Read the model definition and answer for the solid it produces. Units are mm, in the model's axes. A direction names the side the tool comes from. Coordinates: 2 decimals unless noted, no trailing zeros. Loops run counter-clockwise (first coordinate to the right, second up) from the corner with the lowest first, then second, coordinate; pieces in that order, holes last. Notation, with made-up numbers: (-5, 34.25) - (32, 34.25) arc R17 cw to (32, 62.25) - close; hole circle Ø3 at (18, 8.5). An arc over 180 degrees is marked (long way). One line per item, written item: value. Start each with the question number.
Autodesk Inventor part; units mm, degrees
ref_plane "YZ Plane" through (0, 0, 0) normal (1, 0, 0) x (0, 1, 0)
ref_plane "XZ Plane" through (0, 0, 0) normal (0, 1, 0) x (-1, 0, 0)
ref_plane "XY Plane" through (0, 0, 0) normal (0, 0, 1) x (1, 0, 0)
sketch "Sketch1" plane through (0, 0, 0) normal (0, 1, 0) x (-1, 0, 0)
  line L0 (50, 0) -> (0, 0)
  line L1 (0, 0) -> (0, -20)
  line L2 (0, -20) -> (50, -20)
  line L3 (50, -20) -> (50, 0)
  line L4 (0, 0) -> (20, 0)
  line L5 (20, 0) -> (20, -80)
  line L6 (20, -80) -> (0, -80)
  line L7 (0, -80) -> (0, 0)
  point P0 (0, 0)
  point P1 (20, -20)
  dimension "d0" = 50
  dimension "d1" = 20
  dimension "d2" = 80
  dimension "d3" = 20
  dimension "d4" = 0
  dimension "d5" = 0
extrude "Extrusion1" add sketch "Sketch1" along normal blind 10
sketch "Sketch3" plane through (0, 10, 0) normal (0, 1, 0) x (1, 0, 0)
  line L0 (0, 80) -> (-20, 80)
  line L1 (-20, 80) -> (0, 80)
  line L2 (0, 80) -> (0, 72.5)
  line L3 (0, 72.5) -> (-20, 72.5)
  line L4 (-20, 72.5) -> (-20, 80)
  line L5 (0, 0) -> (0, 80)
  line L6 (0, 80) -> (-5, 80)
  line L7 (-5, 80) -> (-5, 0)
  line L8 (-5, 0) -> (0, 0)
  line L9 (0, 0) -> (0, 80)
  line L10 (-50, 20) -> (-50, 0)
  line L11 (0, 0) -> (-50, 0)
  line L12 (0, 10) -> (0, 0)
  line L13 (-50, 0) -> (0, 0)
  line L14 (0, 0) -> (-50, 0)
  line L15 (-50, 0) -> (-50, 5)
  line L16 (-50, 5) -> (0, 5)
  line L17 (0, 5) -> (0, 0)
  point P0 (-50, 10)
  point P1 (-5, 72.5)
  point P2 (-5, 5)
  point P3 (-5, 0)
  dimension "d8" = 20
  dimension "d9" = 7.5
  dimension "d10" = 5
  dimension "d11" = 80
  dimension "d14" = 50
  dimension "d15" = 5
extrude "Extrusion2" add sketch "Sketch3" along normal blind 10 contours L2 L3 L7 L0 | L7 L3 L4 L0 | L5 L16 L7 L3 | L16 L5 L8 L7
extrude "Extrusion3" add sketch "Sketch3" along normal blind 10 contours L7 L11 L10 L16
fillet "Fillet1" radius 2 16 edges at (-5, 20, -38.75) (-5, 10, -38.75) (-27.5, 20, -5) (-27.5, 10, -5) (-5, 15, -5) (-20, 10, -46.25) (-35, 10, -20) (-12.5, 20, -72.5) (-10, 20, -80) (-20, 20, -76.25) (-20, 15, -72.5) (-50, 10, -12.5) (-50, 15, -5) (-50, 20, -2.5) (0, 20, -40) (-25, 20, 0)
sketch "Sketch4" plane through (0, 0, 0) normal (0, -1, 0) x (1, 0, 0)
  line L0 (0, 0) -> (-7.5, 0)
  line L1 (-7.5, 0) -> (-7.5, -7.5)
  line L2 (-7.5, -7.5) -> (0, -7.5)
  line L3 (0, -7.5) -> (0, 0)
  line L4 (-20, -20) -> (-50, -20)
  line L5 (-50, -20) -> (-42.5, -20)
  line L6 (-42.5, -20) -> (-42.5, -12.5)
  line L7 (-42.5, -12.5) -> (-50, -12.5)
  line L8 (-50, -12.5) -> (-50, -20)
  line L9 (-50, 0) -> (0, 0)
  line L10 (-50, 0) -> (-42.5, 0)
  line L11 (-42.5, 0) -> (-42.5, -7.5)
  line L12 (-42.5, -7.5) -> (-50, -7.5)
  line L13 (-50, -7.5) -> (-50, 0)
  line L14 (-18, -18) -> (-20, -20)
  line L15 (-20, -20) -> (-12.3, -20)
  line L16 (-12.3, -20) -> (-12.3, -12.5)
  line L17 (-12.3, -12.5) -> (-20, -12.5)
  line L18 (-20, -12.5) -> (-20, -20)
  line L19 (0, -80) -> (-20, -80)
  line L20 (-20, -80) -> (-12.5, -80)
  line L21 (-12.5, -80) -> (-12.5, -72.5)
  line L22 (-12.5, -72.5) -> (-20, -72.5)
  line L23 (-20, -72.5) -> (-20, -80)
  line L24 (0, 0) -> (0, -80)
  line L25 (0, -80) -> (-7.5, -80)
  line L26 (-7.5, -80) -> (-7.5, -72.5)
  line L27 (-7.5, -72.5) -> (0, -72.5)
  line L28 (0, -72.5) -> (0, -80)
  point P0 (0, -72.5)
  dimension "d19" = 7.5
  dimension "d20" = 7.5
  dimension "d21" = 7.5
  dimension "d22" = 7.5
  dimension "d23" = 7.5
  dimension "d24" = 7.5
  dimension "d25" = 7.7
  dimension "d26" = 7.5
  dimension "d27" = 7.5
  dimension "d28" = 7.5
  dimension "d29" = 7.5
  dimension "d30" = 7.5
extrude "Extrusion4" add sketch "Sketch4" along normal blind 2
properties part number "couch"
1) Flat-ended cylindrical pins translate along their axes: P1, Ø0.6, axis at y = -1.5, z = -15.5, coming from the +X side; P2, Ø12, axis at y = 14.5, z = -18, coming from the -X side; P3, Ø5, axis at x = -21.5, z = -54.5, coming from the -Y side. Find the tip coordinate at first contact, or state that the pin passes through.
2) For faces 1 (the flat face through (-20, -1, -16)), 2 (the flat face through (-35, 4, -20)), 3 (the flat face through (-11, 14, -72.5)), 4 (the cylindrical face through (-49.4, 9.43, -13.41)), determine the directions among +Z, -Z, +X, -X, +Y, -Y from which every point of the face is accessible in a straight line to the end or side of a thin tool.
3) Determine the mould class of faces 5 (the flat face through (-4, -1, -7.5)), 6 (the flat face through (-5, 15, -40)), 7 (the flat face through (-12.5, -1, -76)) for opening direction X: released by +X, released by -X, zero draft, split by the parting line, or undercut.
4) Section A-A, the plane z = -22 is taken. Determine the outline of the cut face in (x, y), and give its area (3 significant figures).
5) Section D-D, the plane y = 2.5 is taken. Determine the outline of the cut face in (x, z).
6) Straight lines are drawn through the part: L1, parallel to Z at x = -31, y = 2.75; L2, parallel to Y at x = -8.5, z = -46; L3, parallel to Z at x = -25.5, y = 18. For each, find the intervals that lie inside material, in ascending order.
7) Section C-C, the plane x = -27.5 is taken. Determine the outline of the cut face in (y, z), and give its area (3 significant figures).
8) Section B-B, the plane y = 15 is taken. Determine the outline of the cut face in (x, z), and give its area (3 significant figures).
Answer below:
1. P1: x = -12.3
1. P2: x = -49.94
1. P3: y = 0
2. face 1: +Z, -Z, -Y
2. face 2: -Z, -X, +Y, -Y
2. face 3: -X, +Y
2. face 4: -Z, -X, +Y
3. face 5: zero draft
3. face 6: released by -X
3. face 7: undercut
4. outline: (-20, 0) - (0, 0) - (0, 18) arc R2 ccw to (-2, 20) - (-3, 20) arc R2 ccw to (-5, 18) - (-5, 12) arc R2 cw to (-7, 10) - (-18, 10) arc R2 ccw to (-20, 8) - close
4. area: 248 mm2
5. outline: (-50, -20) - (-20, -20) - (-20, -80) - (0, -80) - (0, 0) - (-50, 0) - close
6. L1: -20 to 0
6. L2: 0 to 10
6. L3: -5 to 0
7. outline: (0, -20) - (8, -20) arc R2 ccw to (10, -18) - (10, -7) arc R2 cw to (12, -5) - (18, -5) arc R2 ccw to (20, -3) - (20, -2) arc R2 ccw to (18, 0) - (0, 0) - close
7. area: 248 mm2
8. outline: (-50, -3) arc R2 ccw to (-48, -5) - (-7, -5) arc R2 cw to (-5, -7) - (-5, -72.5) - (-18, -72.5) arc R2 ccw to (-20, -74.5) - (-20, -80) - (0, -80) - (0, 0) - (-50, 0) - close
8. area: 737 mm2
